from build123d import *

# Parameters (mm, degrees)
F0_W        = 69.5
F0_H        = 26.3
F1_DEPTH    = 37
F2_W        = 65.5
F2_H        = 22.3
F3_DEPTH    = 35
F4_SIZE     = 0.4
F5_T1_DEPTH = 49.3
F6_R        = 2.54
F7_W        = 8
F7_H        = 4.5
F8_DEPTH    = 1
F9_W        = 7.9342592508
F9_H        = 2.0083109736
F10_DEPTH   = 3
F11_R       = 0.5


# Not quite as in the source:
# - a fillet or chamfer that OpenCascade refuses, or shapes differently, is made with other operations: its cross-section is extruded or revolved along the edge and cut away or added


with BuildPart() as f1:
    # F0 (on Top) → F1 (new body)
    with BuildSketch(Plane.XY):
        Rectangle(F0_W, F0_H)
    extrude(amount=F1_DEPTH)

    # F2 (on face) → F3 (cut)
    with BuildSketch(Plane.XY.offset(37)):
        Rectangle(F2_W, F2_H)
    extrude(amount=-F3_DEPTH, mode=Mode.SUBTRACT)

    # F4
    f4_edges = [f1.edges().sort_by_distance(p)[0] for p in [
        (0, -13.15, 0),
        (34.75, 0, 0),
        (0, 13.15, 0),
        (-34.75, 0, 0),
    ]]
    chamfer(f4_edges, length=F4_SIZE)

    # F5: fillet of radius 2.54 on 4 edges, made by hand

    # F5_s2 → F5_t1 (cut)
    with BuildSketch(Plane.XY.offset(-5.95)):
        with BuildLine():
            ThreePointArc((34.75, 10.61), (34.0060512242, 12.4060512242), (32.21, 13.15))
            Line((32.21, 13.15), (34.75, 13.15))
            Line((34.75, 13.15), (34.75, 10.61))
        make_face()
        with BuildLine():
            ThreePointArc((32.21, -13.15), (34.0060512242, -12.4060512242), (34.75, -10.61))
            Line((34.75, -10.61), (34.75, -13.15))
            Line((34.75, -13.15), (32.21, -13.15))
        make_face()
        with BuildLine():
            ThreePointArc((-34.75, 10.61), (-34.0060512242, 12.4060512242), (-32.21, 13.15))
            Line((-32.21, 13.15), (-34.75, 13.15))
            Line((-34.75, 13.15), (-34.75, 10.61))
        make_face()
        with BuildLine():
            ThreePointArc((-32.21, -13.15), (-34.0060512242, -12.4060512242), (-34.75, -10.61))
            Line((-34.75, -10.61), (-34.75, -13.15))
            Line((-34.75, -13.15), (-32.21, -13.15))
        make_face()
    extrude(amount=F5_T1_DEPTH, mode=Mode.SUBTRACT)

    # F6
    f6_edges = [f1.edges().sort_by_distance(p)[0] for p in [
        (0, -11.15, 2),
        (-32.75, 0, 2),
        (32.75, 0, 2),
        (0, 11.15, 2),
    ]]
    fillet(f6_edges, radius=F6_R)

    # F7 (on face) → F8 (join)
    with BuildSketch(Plane.XZ.offset(-11.15)):
        with Locations((14.25, 34.75)):
            Rectangle(F7_W, F7_H)
    extrude(amount=F8_DEPTH)

    # F9 (on face) → F10 (join)
    with BuildSketch(Plane(origin=(0, 13.15, 0), x_dir=(-1, 0, 0), z_dir=(0, 1, 0))):
        with Locations((-14.2189497128, 35.9958445132)):
            Rectangle(F9_W, F9_H)
    extrude(amount=F10_DEPTH)

    # F11
    f11_edges = [f1.edges().sort_by_distance(p)[0] for p in [
        (32.75, 11.15, 20.77),
        (32.75, -11.15, 20.77),
        (-32.75, -11.15, 20.77),
        (-32.75, 11.15, 20.77),
    ]]
    fillet(f11_edges, radius=F11_R)


solid = f1.part
The model under review builds one solid part; all positions refer to its coordinate system, in mm. A direction names the side the tool comes from. Round coordinates to 2 decimals unless told otherwise and drop trailing zeros. Loops run counter-clockwise (first coordinate to the right, second up) from the corner with the lowest first, then second, coordinate; pieces in that order, holes last. Notation, with made-up numbers: (86, -34.5) -> (111, -34.5) arc R9 ccw to (111, -21.5) -> close; hole circle Ø5 at (-27.5, -6.75). An arc over 180 degrees is marked (long way). Return JSON: item names as keys, results as strings.
(1) Add section A-A on z = 20. Write out the cut boundary in (x, y).
Solved:
{"outline": "(-34.75, -10.61) arc R2.54 ccw to (-32.21, -13.15) -> (32.21, -13.15) arc R2.54 ccw to (34.75, -10.61) -> (34.75, 10.61) arc R2.54 ccw to (32.21, 13.15) -> (-32.21, 13.15) arc R2.54 ccw to (-34.75, 10.61) -> close; hole (-32.75, -10.65) arc R0.5 ccw to (-32.25, -11.15) -> (32.25, -11.15) arc R0.5 ccw to (32.75, -10.65) -> (32.75, 10.65) arc R0.5 ccw to (32.25, 11.15) -> (-32.25, 11.15) arc R0.5 ccw to (-32.75, 10.65) -> close"}
(2) Add section D-D on y = 14. Write out the cut boundary in (x, z), plus the area to 3 significant figures.
Solved:
{"outline": "(10.25, 34.99) -> (18.19, 34.99) -> (18.19, 37) -> (10.25, 37) -> close", "area": "15.9 mm2"}
(3) The part is to be moulded in two halves that separate along Y. For faces 1 (the flat face through (-32.75, 0, 21)), 2 (the flat face through (0, 0, 0)), 3 (the cylindrical face through (34.026, 12.386, 18.241)), 4 (the flat face through (0, -13.15, 18)), say which applies: released by +Y, released by -Y, zero draft, split by the parting line, or undercut.
Solved:
{"face 1": "undercut", "face 2": "zero draft", "face 3": "released by +Y", "face 4": "released by -Y"}
(4) For pin 1 (14 mm diameter, centred on x = 10, y = -3.5, fed in from +Z); pin 2 (1.5 mm diameter, centred on x = 3, y = -0.5, fed in from +Z); pin 3 (3.5 mm diameter, centred on x = 13.5, y = 15, fed in from -Z), all flat-tipped, find the tip position at first contact; note any pin that passes through.
Solved:
{"pin 1": "z = 2.84", "pin 2": "z = 2", "pin 3": "z = 34.99"}
(5) For line 1 (X direction, y = 7.5, z = 29); line 2 (Y direction, x = 21.5, z = 32.5); line 3 (Z direction, x = 29, y = 6.25), list the stretches that pass through material, from the lowest coordinate up.
Solved:
{"line 1": "-34.75 to -32.75, 32.75 to 34.75", "line 2": "-13.15 to -11.15, 11.15 to 13.15", "line 3": "0 to 2"}
(6) For faces 5 (the flat face through (14, 15, 34.992)), 6 (the cylindrical face through (-33.986, -12.426, 18.241)), 7 (the flat face through (18.186, 15, 36)), 8 (the cylindrical face through (33.986, -12.426, 18.241)), 9 (the cylindrical face through (-32.026, 0.149, 2.764)), list the 3-axis set-ups (+Z, -Z, +X, -X, +Y, -Y) from which the entire face can be reached by the end or side of a thin tool; tool diameter is ignored.
Solved:
{"face 5": "-Z, +X, -X, +Y", "face 6": "+Z, -Z, -X, -Y", "face 7": "+Z, -Z, +X, +Y", "face 8": "+Z, -Z, +X, -Y", "face 9": "+Z"}
(7) Add section B-B on x = 29.5. Write out the cut boundary in (y, z), plus the area to 3 significant figures.
Solved:
{"outline": "(-13.15, 0.4) -> (-12.75, 0) -> (12.75, 0) -> (13.15, 0.4) -> (13.15, 37) -> (11.15, 37) -> (11.15, 4.54) arc R2.54 cw to (8.61, 2) -> (-8.61, 2) arc R2.54 cw to (-11.15, 4.54) -> (-11.15, 37) -> (-13.15, 37) -> close", "area": "195 mm2"}
(8) Add section C-C on y = -7.75. Write out the cut boundary in (x, z).
Solved:
{"outline": "(-34.75, 0.4) -> (-34.35, 0) -> (34.35, 0) -> (34.75, 0.4) -> (34.75, 37) -> (32.75, 37) -> (32.75, 4.54) arc R2.54 cw to (30.21, 2) -> (-30.21, 2) arc R2.54 cw to (-32.75, 4.54) -> (-32.75, 37) -> (-34.75, 37) -> close"}
